from build123d import *

# Parameters (mm, degrees)
SKETCH1_R           = 2.125
SKETCH1_W           = 19.725
SKETCH1_H           = 4
BOSS_EXTRUDE1_DEPTH = 4


with BuildPart() as part:
    # Sketch1 → Boss-Extrude1 (new body)
    with BuildSketch(Plane(origin=(0, 0, 0), x_dir=(1, 0, 0), z_dir=(0, 1, 0))):
        with BuildLine():
            Line((4, 0), (4, 20))
            Line((4, 20), (0, 20))
            Line((0, 20), (0, 40))
            Line((0, 40), (4, 40))
            Line((4, 40), (4, 60))
            Line((4, 60), (0, 60))
            Line((0, 60), (0, 80))
            Line((0, 80), (4, 80))
            Line((4, 80), (4, 100))
            Line((4, 100), (250, 100))
            Line((250, 100), (496, 100))
            Line((496, 100), (496, 80))
            Line((496, 80), (500, 80))
            Line((500, 80), (500, 60))
            Line((500, 60), (496, 60))
            Line((496, 60), (496, 40))
            Line((496, 40), (500, 40))
            Line((500, 40), (500, 20))
            Line((500, 20), (496, 20))
            Line((496, 20), (496, 0))
            Line((496, 0), (476, 0))
            Line((476, 0), (476, 5))
            ThreePointArc((476, 5), (456.961940777, 50.961940777), (411, 70))
            Line((411, 70), (89, 70))
            ThreePointArc((89, 70), (43.038059223, 50.961940777), (24, 5))
            Line((24, 5), (24, 0))
            Line((24, 0), (4, 0))
        make_face()
        with Locations((14, 15)):
            Circle(SKETCH1_R, mode=Mode.SUBTRACT)
        with Locations((14, 30)):
            Circle(SKETCH1_R, mode=Mode.SUBTRACT)
        with Locations((173.885, 90)):
            Circle(SKETCH1_R, mode=Mode.SUBTRACT)
        with Locations((326.115, 90)):
            Circle(SKETCH1_R, mode=Mode.SUBTRACT)
        with Locations((486, 30)):
            Circle(SKETCH1_R, mode=Mode.SUBTRACT)
        with Locations((486, 15)):
            Circle(SKETCH1_R, mode=Mode.SUBTRACT)
        with Locations((14, 60)):
            Circle(SKETCH1_R, mode=Mode.SUBTRACT)
        with Locations((14, 45)):
            Circle(SKETCH1_R, mode=Mode.SUBTRACT)
        with Locations((486, 45)):
            Circle(SKETCH1_R, mode=Mode.SUBTRACT)
        with Locations((486, 60)):
            Circle(SKETCH1_R, mode=Mode.SUBTRACT)
        with Locations((63.3125, 78)):
            Rectangle(SKETCH1_W, SKETCH1_H, mode=Mode.SUBTRACT)
        with Locations((23.8625, 78)):
            Rectangle(SKETCH1_W, SKETCH1_H, mode=Mode.SUBTRACT)
        with Locations((102.7625, 78)):
            Rectangle(SKETCH1_W, SKETCH1_H, mode=Mode.SUBTRACT)
        with Locations((142.2125, 78)):
            Rectangle(SKETCH1_W, SKETCH1_H, mode=Mode.SUBTRACT)
        with Locations((181.6625, 78)):
            Rectangle(SKETCH1_W, SKETCH1_H, mode=Mode.SUBTRACT)
        with Locations((221.1125, 78)):
            Rectangle(SKETCH1_W, SKETCH1_H, mode=Mode.SUBTRACT)
        with Locations((278.8875, 78)):
            Rectangle(SKETCH1_W, SKETCH1_H, mode=Mode.SUBTRACT)
        with Locations((318.3375, 78)):
            Rectangle(SKETCH1_W, SKETCH1_H, mode=Mode.SUBTRACT)
        with Locations((357.7875, 78)):
            Rectangle(SKETCH1_W, SKETCH1_H, mode=Mode.SUBTRACT)
        with Locations((397.2375, 78)):
            Rectangle(SKETCH1_W, SKETCH1_H, mode=Mode.SUBTRACT)
        with Locations((436.6875, 78)):
            Rectangle(SKETCH1_W, SKETCH1_H, mode=Mode.SUBTRACT)
        with Locations((476.1375, 78)):
            Rectangle(SKETCH1_W, SKETCH1_H, mode=Mode.SUBTRACT)
    extrude(amount=BOSS_EXTRUDE1_DEPTH)


solid = part.part
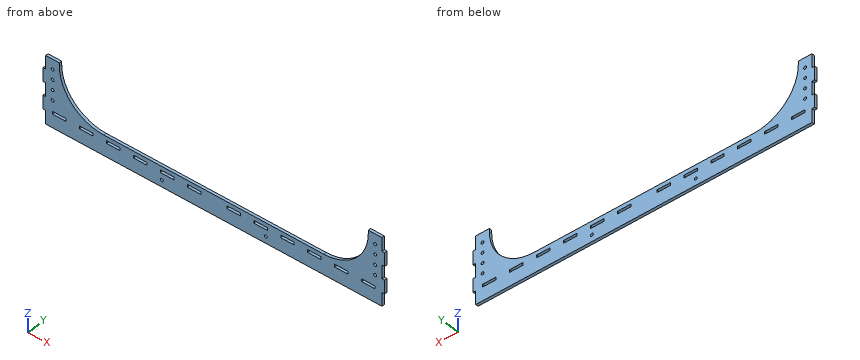
Verification items for the finished model (mm, model axes). Coordinates: 2 decimals unless noted, no trailing zeros. Order: outer loops, then holes, each group sorted by start corner. A loop starts at its lowest first (then second) coordinate and runs counter-clockwise, first axis right, second up. Notation, with made-up numbers: M -14,12.25 L 12,12.25 A13 cw 12,23.25 Z; hole C -28,61.25 d8. An arc over 180 degrees is marked long. One line per item, written item: value. Start each with the question number.
Item 1: Sectioned sample at C-C on x = 459.5. Record the cut outline in (y, z).
Item 2: Thickness scan on probe 1 along X at (y, z) = (1.2, -90); probe 2 along X at (y, z) = (2.75, -45.5); probe 3 along Z at (x, y) = (269.5, 2.85). Record the ranges inside material, lowest first.
Item 3: Sectioned sample at B-B on y = 2.6. Give the number of separate pieces and of enclosed holes in the cut face, then the cut area to 3 significant figures.
Item 4: Sectioned sample at A-A on x = 343.5. Record the cut outline in (y, z).
Item 5: Depth check by flat-ended pin: P1, Ø2, axis at x = 270, y = 2, coming from the +Z side; P2, Ø1.5, axis at x = 56, y = 3.5, coming from the +Z side; P3, Ø2, axis at x = 1.5, y = 2.5, coming from the -Z side. Enter the tip coordinate at first touch or a pass-through.
Calculated:
1. outline: M 0,-100 L 4,-100 L 4,-48.28 L 0,-48.28 Z
2. probe 1: 4 to 171.76, 176.01 to 323.99, 328.24 to 496
2. probe 2: 4 to 11.93, 16.07 to 38.16, 461.84 to 483.93, 488.07 to 496
2. probe 3: -100 to -80, -76 to -70
3. separate pieces: 1
3. enclosed holes: 22
3. area: 18,600 mm^2
4. outline: M 0,-100 L 4,-100 L 4,-70 L 0,-70 Z
5. P1: z = -70
5. P2: z = -60.55
5. P3: z = -80
